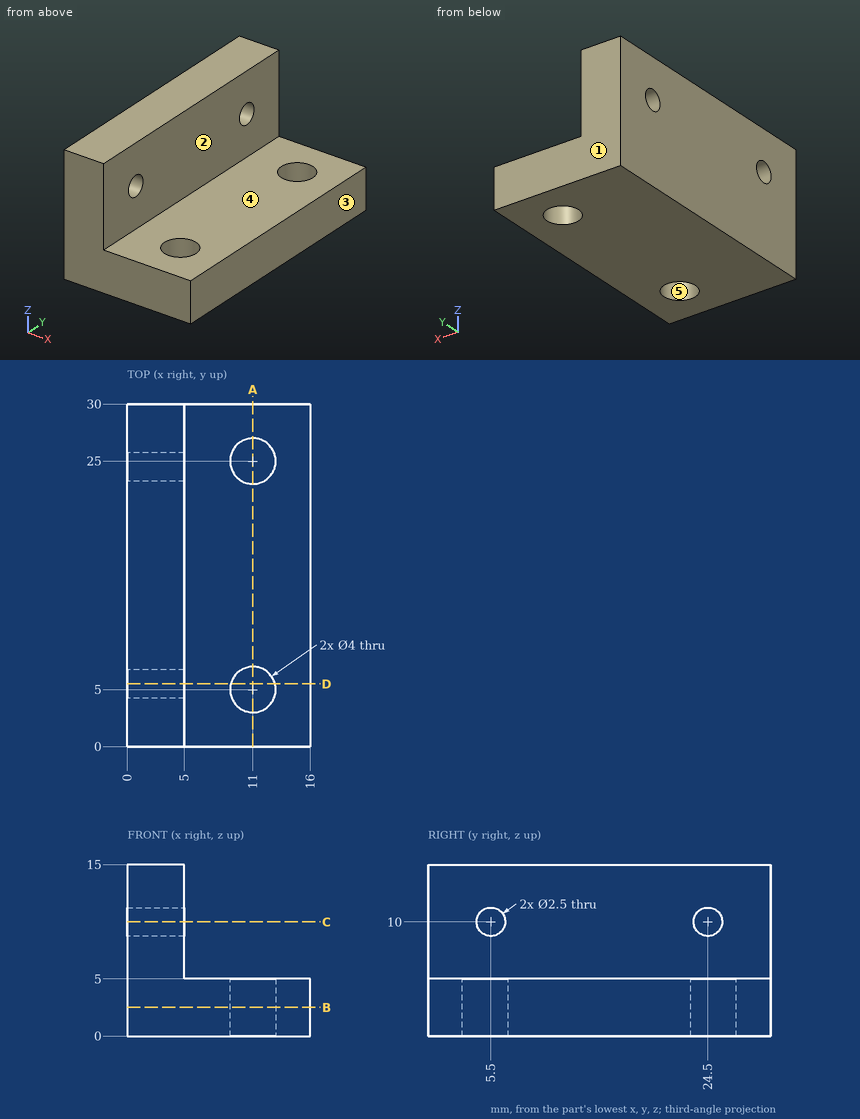
Geometry check sheet. Reference: drawing and pictorial views, mm from the part's lowest x, y, z. A direction names the side the tool comes from. Coordinates: 2 decimals unless noted, no trailing zeros. Order: outer loops, then holes, each group sorted by start corner. A loop starts at its lowest first (then second) coordinate and runs counter-clockwise, first axis right, second up. Notation, with made-up numbers: M 80,45 L 98,45 A30 cw 98,71 Z; hole C 60,1 d7. An arc over 180 degrees is marked long. Return JSON: item names as keys, results as strings.
1) Thickness scan on L1, parallel to Y at x = 3.45, z = 10; L2, parallel to Y at x = 11, z = 2.75; L3, parallel to Z at x = 9.25, y = 10.25. Record the ranges inside material, lowest first. Write a range as [from, to].
Answer list:
{"L1": "[0, 4.25], [6.75, 23.25], [25.75, 30]", "L2": "[0, 3], [7, 23], [27, 30]", "L3": "[0, 5]"}
2) Gauge pin test, flat ends, axial feed: pin 1 (3.5 mm diameter, centred on x = 11, y = 25, fed in from +Z); pin 2 (4 mm diameter, centred on x = 11.5, y = 17, fed in from +Z); pin 3 (8 mm diameter, centred on y = 17.5, z = 12, fed in from +X). Record the tip position at first contact, or that the pin passes through.
Answer list:
{"pin 1": "through", "pin 2": "z = 5", "pin 3": "x = 5"}
3) Release check for a two-part mould opening along X. For the marked faces 3, 4 and 5 record: +X half, -X half, draft (parallel to the pull), parting line (faces both ways), or undercut.
Answer list:
{"face 3": "+X half", "face 4": "draft", "face 5": "undercut"}
4) Access from +Z, -Z, +X, -X, +Y, -Y to the whole of each face (thin tool, end or side, straight path). Record for the marked faces 1 and 2.
Answer list:
{"face 1": "+Z, -Z, +X, -X, +Y", "face 2": "+Z, +X, +Y, -Y"}
5) Cross-section at B-B, the plane z = 2.5. Record the boundary of the cut face in (x, y).
Answer list:
{"outline": "M 0,0 L 16,0 L 16,30 L 0,30 Z; hole C 11,5 d4; hole C 11,25 d4"}
6) Cross-section at A-A, the plane x = 11. Record the boundary of the cut face in (y, z).
Answer list:
{"outline": "M 0,0 L 3,0 L 3,5 L 0,5 Z; M 7,0 L 23,0 L 23,5 L 7,5 Z; M 27,0 L 30,0 L 30,5 L 27,5 Z"}
7) Cross-section at C-C, the plane z = 10. Record the boundary of the cut face in (x, y), and give its area (3 significant figures).
Answer list:
{"outline": "M 0,0 L 5,0 L 5,4.25 L 0,4.25 Z; M 0,6.75 L 5,6.75 L 5,23.25 L 0,23.25 Z; M 0,25.75 L 5,25.75 L 5,30 L 0,30 Z", "area": "125 mm2"}
8) Cross-section at D-D, the plane y = 5.5. Record the boundary of the cut face in (x, z).
Answer list:
{"outline": "M 0,0 L 9.06,0 L 9.06,5 L 5,5 L 5,8.75 L 0,8.75 Z; M 0,11.25 L 5,11.25 L 5,15 L 0,15 Z; M 12.94,0 L 16,0 L 16,5 L 12.94,5 Z"}
